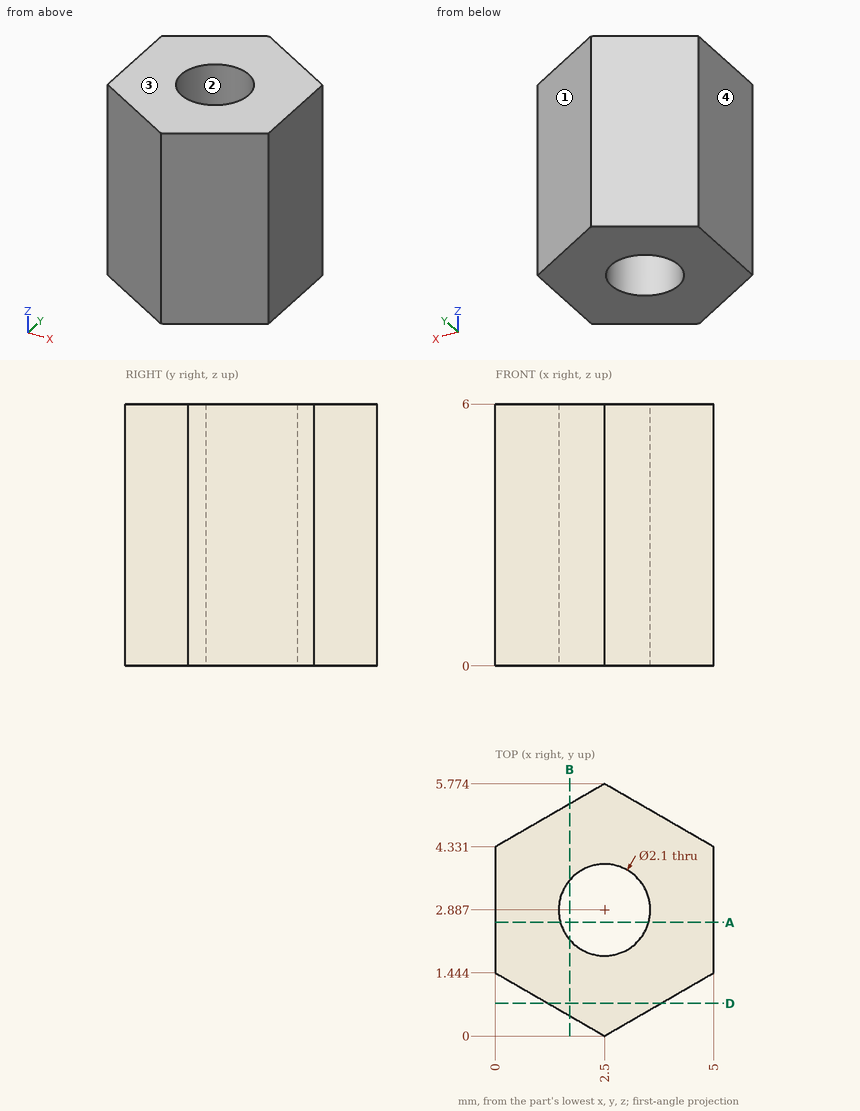
Verification items for this drawing (mm, ordinates from the low corner). Give positions to 0.01 mm unless a question says otherwise; leave off trailing zeros. Loops run counter-clockwise (first coordinate to the right, second up) from the corner with the lowest first, then second, coordinate; pieces in that order, holes last. Notation, with made-up numbers: M -36.5,-15 L -5.5,-15 A9 ccw -5.5,-11 Z; hole C 79.25,25.5 d5. An arc over 180 degrees is marked long. Write item = value, one per line. Start each with the question number.
1. Thickness scan on probe 1 along X at (y, z) = (3.3, 3.1) (1 decimal); probe 2 along X at (y, z) = (2.25, 4.65) (1 decimal); probe 3 along Y at (x, z) = (2.05, 1.9) (1 decimal). Record the ranges inside material, lowest first.
2. Draft check along X on the marked faces 1, 2, 3 and 4. Enter one of: +X half, -X half, draft (parallel to the pull), parting line (faces both ways), or undercut.
3. Go/stop test with a flat-tipped pin: P1, Ø1.5, axis at x = 4, z = 3, coming from the +Y side. Record where the tip stops, or that it passes through.
4. Section check D-D, the plane y = 0.75. Enter the section's corners in (x, z), plus the area to 3 significant figures.
5. Section check A-A, the plane y = 2.6. Enter the section's corners in (x, z).
6. Section check B-B, the plane x = 1.7. Enter the section's corners in (y, z).
Values follow:
q1.probe_1 = 0 to 1.5, 3.5 to 5
q1.probe_2 = 0 to 1.7, 3.3 to 5
q1.probe_3 = 0.3 to 1.9, 3.8 to 5.5
q2.face_1 = +X half
q2.face_2 = undercut
q2.face_3 = draft
q2.face_4 = -X half
q3.P1 = 5.34
q4.outline = M 1.2,0 L 3.8,0 L 3.8,6 L 1.2,6 Z
q4.area = 15.6 mm^2
q5.outline = M 0,0 L 1.49,0 L 1.49,6 L 0,6 Z; M 3.51,0 L 5,0 L 5,6 L 3.51,6 Z
q6.outline = M 0.46,0 L 2.21,0 L 2.21,6 L 0.46,6 Z; M 3.57,0 L 5.31,0 L 5.31,6 L 3.57,6 Z
